```python
from build123d import *

# Parameters (mm, degrees)
SKETCH_W           = 8.8
SKETCH_H           = 11.8
PAD_DEPTH          = 4.48
FILLET_R           = 1
SKETCH001_R        = 0.85
PAD001_DEPTH       = 1
FILLET001_R        = 0.6
SKETCH002_R        = 3
PAD002_DEPTH       = 23
CHAMFER_SIZE       = 0.3
POCKET_DEPTH       = 7
POLARPATTERN_COUNT = 25
SKETCH004_R        = 0.8
SKETCH004_R_2      = 0.65
PAD003_DEPTH       = 1.5
CHAMFER001_SIZE    = 0.3
SKETCH010_W        = 4
SKETCH010_H        = 1.5
POCKET004_DEPTH    = 2.5


with BuildPart() as part:
    # Sketch → Pad (new body)
    with BuildSketch(Plane.XY):
        with Locations((0, -0.4)):
            Rectangle(SKETCH_W, SKETCH_H)
    extrude(amount=-PAD_DEPTH)

    # Fillet
    fillet_edges = [part.edges().sort_by_distance(p)[0] for p in [
        (-4.4, 5.5, -2.24),
        (-4.4, -6.3, -2.24),
        (4.4, -6.3, -2.24),
        (4.4, 5.5, -2.24),
    ]]
    fillet(fillet_edges, radius=FILLET_R)

    # Sketch001 (on Face2 of Fillet) → Pad001 (join)
    with BuildSketch(Plane.XY):
        with Locations((-3, 4.2)):
            Circle(SKETCH001_R)
        with Locations((3, 4.2)):
            Circle(SKETCH001_R)
        with Locations((3, -4.2)):
            Circle(SKETCH001_R)
        with Locations((-3, -4.2)):
            Circle(SKETCH001_R)
    extrude(amount=PAD001_DEPTH)

    # Fillet001
    fillet001_edges = [part.edges().sort_by_distance(p)[0] for p in [
        (-3.85, -4.2, 1),
        (-3.85, 4.2, 1),
        (2.15, 4.2, 1),
        (2.15, -4.2, 1),
    ]]
    fillet(fillet001_edges, radius=FILLET001_R)

    # Sketch002 (on Face3 of Fillet001) → Pad002 (join)
    with BuildSketch(Plane.XY):
        Circle(SKETCH002_R)
    extrude(amount=PAD002_DEPTH)

    # Chamfer
    chamfer_edges = [part.edges().sort_by_distance(p)[0] for p in [
        (-3, 0, 23),
    ]]
    chamfer(chamfer_edges, length=CHAMFER_SIZE)

    # Sketch003 (on Face20 of Pad002) → Pocket (cut)
    with BuildSketch(Plane.XY.offset(23)):
        Polygon((-0.55, 3.1), (0, 2.6), (0.55, 3.1), align=None)
    pocket = extrude(amount=-POCKET_DEPTH, mode=Mode.SUBTRACT)

    # PolarPattern: Pocket ×25 about axis
    polarpattern_axis = Axis((0, 0, 23), (0, 0, 1))
    for i in range(1, POLARPATTERN_COUNT):
        add(pocket.rotate(polarpattern_axis, i * 360 / POLARPATTERN_COUNT), mode=Mode.SUBTRACT)

    # Sketch004 (on Face126 of PolarPattern) → Pad003 (join)
    with BuildSketch(Plane(origin=(0, 0, -4.48), x_dir=(1, 0, 0), z_dir=(0, 0, -1))):
        with Locations((-3, 4.2)):
            Circle(SKETCH004_R)
        with Locations((3, 4.2)):
            Circle(SKETCH004_R)
        with Locations((3, -4.2)):
            Circle(SKETCH004_R)
        with Locations((-3, -4.2)):
            Circle(SKETCH004_R)
        with Locations((0, -4.2)):
            Circle(SKETCH004_R_2)
        with Locations((0, 4.2)):
            Circle(SKETCH004_R_2)
    extrude(amount=PAD003_DEPTH)

    # Chamfer001
    chamfer001_edges = [part.edges().sort_by_distance(p)[0] for p in [
        (2.2, -4.2, -5.98),
        (-0.65, -4.2, -5.98),
        (-3.8, -4.2, -5.98),
        (-3.8, 4.2, -5.98),
        (-0.65, 4.2, -5.98),
        (2.2, 4.2, -5.98),
    ]]
    chamfer(chamfer001_edges, length=CHAMFER001_SIZE)

    # Sketch010 (on Face12 of Chamfer001) → Pocket004 (cut)
    with BuildSketch(Plane.XZ.offset(6.3)):
        with Locations((0, -0.75)):
            Rectangle(SKETCH010_W, SKETCH010_H)
    extrude(amount=-POCKET004_DEPTH, mode=Mode.SUBTRACT)


solid = part.part
```
Geometry check sheet. Reference: the model listing, model coordinates, mm. A direction names the side the tool comes from. Give positions to 0.01 mm unless a question says otherwise; leave off trailing zeros. Order: outer loops, then holes, each group sorted by start corner. A loop starts at its lowest first (then second) coordinate and runs counter-clockwise, first axis right, second up.
1. Access from +Z, -Z, +X, -X, +Y, -Y to the whole of each face (thin tool, end or side, straight path). Record for faces 1 (the face through (-3, 0, 8)), 2 (the face through (4.4, 0, -2)), 3 (the face through (-3, -4, -5.98)), 4 (the face through (2, -5, -1)), 5 (the face through (3.37, -3.49, -5.07)).
2. Thickness scan on L1, parallel to Z at x = -1, y = -2.75; L2, parallel to Z at x = -2.5, y = -5; L3, parallel to X at y = 1.5, z = 8.25. Record the ranges inside material, lowest first.
3. Gauge pin test, flat ends, axial feed: pin 1 Ø2 at (x, z) = (1, 2) entering from -Y; pin 2 Ø5 at (y, z) = (4, 13) entering from +X; pin 3 Ø2 at (y, z) = (2.5, 8) entering from -X. Record the tip position at first contact, or that the pin passes through.
4. Release check for a two-part mould opening along X. For faces 6 (the face through (-3, 4, -5.98)), 7 (the face through (2.4, -3.6, 0.2)), 8 (the face through (4.115, 5.199, -2.271)) record: pulls with the +X half, pulls with the -X half, needs draft (parallel to the pull), parting line crosses it, or undercut.
5. Section check A-A, the plane z = 13.5. Enter the section's corners in (x, y), and give its area (3 significant figures).
Values follow:
1. face 1: +Z
1. face 2: +Z, -Z, +X, +Y, -Y
1. face 3: -Z, +X, -X, +Y, -Y
1. face 4: +Z, -Y
1. face 5: -Z
2. L1: z = -4.48 to 16
2. L2: z = -4.48 to 0
2. L3: x = -2.6 to 2.6
3. pin 1: stops at y = -3
3. pin 2: stops at x = 2.6
3. pin 3: stops at x = -2.6
4. face 6: needs draft
4. face 7: undercut
4. face 8: pulls with the +X half
5. outline: circle Ø6 at (0, 0)
5. area: 28.3 mm2
